Input: part model. Units: mm. Frame: model coordinates. A direction names the side the tool comes from. Round coordinates to 2 decimals unless told otherwise and drop trailing zeros. Loops run counter-clockwise (first coordinate to the right, second up) from the corner with the lowest first, then second, coordinate; pieces in that order, holes last. Notation, with made-up numbers: (59, 54) - (66, 54) arc R25 cw to (66, 67) - close; hole circle Ø3 at (35.5, 58.25). An arc over 180 degrees is marked (long way). Use CSV: the item, a comma, the result in double quotes. Start each with the question number.
1. Cut plane C-C (x = -7). Return loops of the section in (y, z).
2. Access query for faces 5 (the flat face through (29.265, -7.111, 5.07)), 6 (the flat face through (40.061, -40, 5)), 7 (the flat face through (19, 40.123, 5)), 8 (the flat face through (53, -48.877, 5)), 9 (the flat face through (66.561, -2, 5)). Directions: +Z, -Z, +X, -X, +Y, -Y. A direction counts if a zero-diameter tool reaches every point of the face in a straight line with its end or side. Return the directions, or none.
3. Cut plane B-B (y = -4.5). Return loops of the section in (x, z).
4. Cut plane D-D (z = 7). Return loops of the section in (x, y).
5. Pin query (flat end, axial travel): P1, Ø3, axis at y = -25, z = 8, coming from the -X side; P2, Ø3, axis at x = 34, z = 6.5, coming from the -Y side; P3, Ø2, axis at x = 15, z = 2.5, coming from the -Y side; P4, Ø10.5, axis at x = -21, y = 37.74, coming from the -Z side. Return the tip coordinate at first contact, or that it passes through.
6. Material intervals for probe 1 along X at (y, z) = (18, 5.5); probe 2 along X at (y, z) = (42.5, 6.5); probe 3 along Y at (x, z) = (55, 8.5), sorted ascending. Write a range as from..to.
7. Cut plane A-A (y = 30). Return loops of the section in (x, z), and give its area (3 significant figures).
8. Pull-direction query (Y, two-part tool) for faces 1 (the flat face through (30, 34.742, 5)), 2 (the flat face through (6.989, -5.305, 5.07)), 3 (the flat face through (50.249, 43, 5)), 4 (the cylindrical face through (50.198, -22.896, 4.93)); classes: +Y half, -Y half, draft (parallel to the pull), parting line (faces both ways), or undercut.
```python
from build123d import *

# Parameters (mm, degrees)
F0_W      = 100.584
F0_H      = 98
F1_DEPTH  = 10
F3_D      = 6.528
F4_W      = 60.96
F4_H      = 6
F5_DEPTH  = 10
F7_DEPTH  = 10
F10_DEPTH = 10
F9_W      = 3.5
F9_H      = 98
F11_DEPTH = 10
F12_D     = 6.528
F13_W     = 26.5
F13_H     = 3
F14_DEPTH = 10
F16_DEPTH = 10


with BuildPart() as f1:
    # F0 (on Top) → F1 (new body)
    with BuildSketch(Plane.XY):
        with Locations((19.76898, -2.876867)):
            Rectangle(F0_W, F0_H)
    extrude(amount=F1_DEPTH)

    # F3 (through all)
    with Locations(Plane.XY.offset(10)):
        with Locations((-20.99802, 37.741133), (60.53598, 37.741133)):
            Hole(F3_D / 2)

    # F4 (on face) → F5 (cut, through all)
    with BuildSketch(Plane.XY.offset(10)):
        with Locations((19.76898, 43.123133)):
            Rectangle(F4_W, F4_H)
    extrude(amount=-F5_DEPTH, mode=Mode.SUBTRACT)

    # F6 (on face) → F7 (cut, through all)
    with BuildSketch(Plane.XY.offset(10)):
        Polygon((-30.52302, -51.876867), (40.06098, -51.876867), (40.06098, -30.325267), (-30.52302, 23.072742), align=None)
    extrude(amount=-F7_DEPTH, mode=Mode.SUBTRACT)

    # F9 (on face) → F10 (cut, through all)
    with BuildSketch(Plane.XY.offset(10)):
        Polygon((-30.52302, 23.072742), (-27.02302, 20.424932), (-27.02302, 46.123133), (-30.52302, 46.123133), align=None)
    extrude(amount=-F10_DEPTH, mode=Mode.SUBTRACT)

    # F9 (on face) → F11 (cut, through all)
    with BuildSketch(Plane.XY.offset(10)):
        with Locations((68.31098, -2.876867)):
            Rectangle(F9_W, F9_H)
    extrude(amount=-F11_DEPTH, mode=Mode.SUBTRACT)

    # F12 (through all)
    with Locations(Plane.XY.offset(10)):
        with Locations((53.31098, 20.323133), (53.31098, -43.876867), (53.31098, -23.876867)):
            Hole(F12_D / 2)

    # F13 (on face) → F14 (cut, through all)
    with BuildSketch(Plane.XY.offset(10)):
        with Locations((53.31098, -50.376867)):
            Rectangle(F13_W, F13_H)
    extrude(amount=-F14_DEPTH, mode=Mode.SUBTRACT)

    # F15 (on face) → F16 (cut, through all)
    with BuildSketch(Plane.XY.offset(10)):
        Polygon((10.423962, 34.742446), (-10.100968, 34.742446), (-10.100968, 22.670163), (10.423962, 7.1427), align=None)
        Polygon((38.931154, 34.742446), (19.865519, 34.742446), (19.865519, 0), (38.931154, -14.423481), align=None)
    extrude(amount=-F16_DEPTH, mode=Mode.SUBTRACT)


solid = f1.part
```
Established:
1,outline,"(5.28, 0) - (20.32, 0) - (20.32, 10) - (5.28, 10) - close; (34.74, 0) - (40.12, 0) - (40.12, 10) - (34.74, 10) - close"
2,face 5,"+Z, -Z"
2,face 6,"+Z, -Z, -X, -Y"
2,face 7,"+Z, -Z, +Y"
2,face 8,"+Z, -Z, +X, -X, -Y"
2,face 9,"+Z, -Z, +X, +Y, -Y"
3,outline,"(5.92, 0) - (25.81, 0) - (25.81, 10) - (5.92, 10) - close; (38.93, 0) - (66.56, 0) - (66.56, 10) - (38.93, 10) - close"
4,outline,"(-27.02, 20.42) - (40.06, -30.33) - (40.06, -48.88) - (66.56, -48.88) - (66.56, 46.12) - (50.25, 46.12) - (50.25, 40.12) - (-10.71, 40.12) - (-10.71, 46.12) - (-27.02, 46.12) - close; hole circle Ø6.53 at (-21, 37.74); hole (-10.1, 22.67) - (10.42, 7.14) - (10.42, 34.74) - (-10.1, 34.74) - close; hole (19.87, 0) - (38.93, -14.42) - (38.93, 34.74) - (19.87, 34.74) - close; hole circle Ø6.53 at (53.31, -43.88); hole circle Ø6.53 at (53.31, -23.88); hole circle Ø6.53 at (53.31, 20.32); hole circle Ø6.53 at (60.54, 37.74)"
5,P1,"stops at x = 31.04"
5,P2,"stops at y = -26.87"
5,P3,"stops at y = -12.12"
5,P4,"stops at z = 0"
6,probe 1,"x = -23.82..-3.93, 10.42..19.87, 38.93..51.02, 55.6..66.56"
6,probe 2,"x = -27.02..-10.71, 50.25..66.56"
6,probe 3,"y = -48.88..-46.67, -41.08..-26.67, -21.08..17.53, 23.12..46.12"
7,outline,"(-27.02, 0) - (-10.1, 0) - (-10.1, 10) - (-27.02, 10) - close; (10.42, 0) - (19.87, 0) - (19.87, 10) - (10.42, 10) - close; (38.93, 0) - (66.56, 0) - (66.56, 10) - (38.93, 10) - close"
7,area,"540 mm2"
8,face 1,"undercut"
8,face 2,"-Y half"
8,face 3,"draft"
8,face 4,"undercut"
